from build123d import *

# Parameters (mm, degrees)
F0_R     = 15
F1_DEPTH = 5


with BuildPart() as f1:
    # F0 (on Top) → F1 (new body)
    with BuildSketch(Plane.XY):
        with BuildLine():
            Line((35.638593, 10), (-50, 10))
            Line((-50, 10), (-50, -10))
            Line((-50, -10), (35.638593, -10))
            ThreePointArc((35.638593, -10), (32.5, 0), (35.638593, 10))
        make_face()
        with BuildLine():
            ThreePointArc((67.5, 0), (55.240486, 16.696925), (35.638593, 10))
            ThreePointArc((35.638593, 10), (32.5, 0), (35.638593, -10))
            ThreePointArc((35.638593, -10), (55.240486, -16.696925), (67.5, 0))
        make_face()
        with Locations((50, 0)):
            Circle(F0_R, mode=Mode.SUBTRACT)
    extrude(amount=F1_DEPTH)


solid = f1.part
Geometry: final body of the model. Coordinates: model frame, mm. A direction names the side the tool comes from. Give positions to 0.01 mm unless a question says otherwise; leave off trailing zeros. Order: outer loops, then holes, each group sorted by start corner. A loop starts at its lowest first (then second) coordinate and runs counter-clockwise, first axis right, second up. Notation, with made-up numbers: (8.25, 23) -> (66.25, 23) arc R19 ccw to (66.25, 28) -> close; hole circle Ø6 at (41, 58.5). An arc over 180 degrees is marked (long way). Answer as a JSON object with one key per item and string values.
Q1. Section D-D (x = 2). Output: boundary loops of the cut face in (y, z), plus the area to 3 significant figures.
Entries:
{"outline": "(-10, 0) -> (10, 0) -> (10, 5) -> (-10, 5) -> close", "area": "100 mm^2"}
Q2. Section B-B (z = 1.3). Output: boundary loops of the cut face in (x, y), plus the area to 3 significant figures.
Entries:
{"outline": "(-50, -10) -> (35.64, -10) arc R17.5 ccw (long way) to (35.64, 10) -> (-50, 10) -> close; hole circle Ø30 at (50, 0)", "area": "1,930 mm^2"}
Q3. Draft query along Y for faces 1 (the flat face through (-5, 0, 5)), 2 (the cylindrical face through (35.015, 0.66, 2.465)), 3 (the flat face through (-8, -10, 2)). Return one class per face: released by +Y, released by -Y, zero draft, split by the parting line, or undercut.
Entries:
{"face 1": "zero draft", "face 2": "undercut", "face 3": "released by -Y"}
Q4. Section C-C (y = -2.5). Output: boundary loops of the cut face in (x, z).
Entries:
{"outline": "(-50, 0) -> (35.21, 0) -> (35.21, 5) -> (-50, 5) -> close; (64.79, 0) -> (67.32, 0) -> (67.32, 5) -> (64.79, 5) -> close"}
Q5. Section A-A (x = 50). Output: boundary loops of the cut face in (y, z).
Entries:
{"outline": "(-17.5, 0) -> (-15, 0) -> (-15, 5) -> (-17.5, 5) -> close; (15, 0) -> (17.5, 0) -> (17.5, 5) -> (15, 5) -> close"}
Q6. Access query for faces 4 (the flat face through (-7, 10, 2)), 5 (the flat face through (-5, 0, 0)). Directions: +Z, -Z, +X, -X, +Y, -Y. A direction counts if a zero-diameter tool reaches every point of the face in a straight line with its end or side. Return the directions, or none.
Entries:
{"face 4": "+Z, -Z, -X, +Y", "face 5": "-Z, +X, -X, +Y, -Y"}
Q7. First-contact query: pin 1 (2 mm diameter, centred on x = 7, z = 3.5, fed in from +Y); pin 2 (1 mm diameter, centred on x = -29, z = 4.5, fed in from -Y). Flat tips, straight axial feed; report the tip coordinate or a pass-through.
Entries:
{"pin 1": "stops at y = 10", "pin 2": "stops at y = -10"}
Q8. Material intervals for probe 1 along Y at (x, z) = (50, 2.2); probe 2 along Y at (x, z) = (-12, 2.5); probe 3 along X at (y, z) = (8, 3.55), sorted ascending.
Entries:
{"probe 1": "y = -17.5 to -15, 15 to 17.5", "probe 2": "y = -10 to 10", "probe 3": "x = -50 to 37.31, 62.69 to 65.56"}
